Geometry: final body of the model. Coordinates: model frame, mm. Give positions to 0.01 mm unless a question says otherwise; leave off trailing zeros. Write each loop counter-clockwise with the first axis right and the second up, starting at its lowest first coordinate (ties: lowest second). Pieces come first, ordered by that corner, then holes. Notation, with made-up numbers: M 54.25,-12 L 77.25,-12 A22 ccw 77.25,1 Z; hole C -21.75,35.25 d2. An arc over 180 degrees is marked long. Answer as a JSON object with one key per item and string values.
from build123d import *

# Parameters (mm, degrees)
F0_W     = 140
F0_H     = 25
F1_DEPTH = 5
F2_W     = 137.275629
F2_H     = 21.727344
F4_DEPTH = 2
F3_W     = 137.275629
F3_H     = 21.727344
F3_W_2   = 135.43924
F3_H_2   = 19.634312
F5_DEPTH = 2


with BuildPart() as f1:
    # F0 (on Top) → F1 (new body)
    with BuildSketch(Plane.XY):
        with Locations((25.895725, -23.401141)):
            Rectangle(F0_W, F0_H)
    extrude(amount=F1_DEPTH)

    # F2 (on face) → F4 (cut)
    with BuildSketch(Plane.XY.offset(5)):
        with Locations((25.771517, -23.499948)):
            Rectangle(F2_W, F2_H)
    extrude(amount=F4_DEPTH, mode=Mode.SUBTRACT)

    # F3 (on face) → F5 (cut)
    with BuildSketch(Plane.XY.offset(5)):
        with Locations((25.771517, -23.499948)):
            Rectangle(F3_W, F3_H)
        with Locations((25.588829, -23.667381)):
            Rectangle(F3_W_2, F3_H_2, mode=Mode.SUBTRACT)
    extrude(amount=-F5_DEPTH, mode=Mode.SUBTRACT)


solid = f1.part
1) Cut plane A-A on z = 4.2. Return loops of the section in (x, y).
Geometry check:
{"outline": "M -44.1,-35.9 L 95.9,-35.9 L 95.9,-10.9 L -44.1,-10.9 Z; M -42.13,-33.48 L 93.31,-33.48 L 93.31,-13.85 L -42.13,-13.85 Z; hole M -42.87,-34.36 L 94.41,-34.36 L 94.41,-12.64 L -42.87,-12.64 Z"}
2) Cut plane B-B on x = 85. Return loops of the section in (y, z), and give its area (3 significant figures).
Geometry check:
{"outline": "M -35.9,0 L -10.9,0 L -10.9,5 L -12.64,5 L -12.64,3 L -13.85,3 L -13.85,5 L -33.48,5 L -33.48,3 L -34.36,3 L -34.36,5 L -35.9,5 Z", "area": "121 mm2"}
3) Line query: line 1 (X direction, y = -23.25, z = 3.6); line 2 (Y direction, x = 28.5, z = 3.1). Output: solid intervals per line, ascending. Write a range as from..to.
Geometry check:
{"line 1": "x = -44.1..-42.87, -42.13..93.31, 94.41..95.9", "line 2": "y = -35.9..-34.36, -33.48..-13.85, -12.64..-10.9"}
4) Pull-direction query (X, two-part tool) for faces 1 (the flat face through (25, -35.901, 2)), 2 (the flat face through (-44.104, -24, 2)), 3 (the flat face through (25, -13, 3)); classes: pulls with the +X half, pulls with the -X half, needs draft (parallel to the pull), parting line crosses it, or undercut.
Geometry check:
{"face 1": "needs draft", "face 2": "pulls with the -X half", "face 3": "undercut"}
